from build123d import *

# Parameters (mm, degrees)
SKETCH1_R           = 10
BOSS_EXTRUDE1_DEPTH = 61
SKETCH3_W           = 66
SKETCH3_H           = 1.5
SKETCH4_W           = 45
SKETCH4_H           = 1.5
SKETCH5_W           = 25
SKETCH5_H           = 2.5
SKETCH6_W           = 39.5
SKETCH6_H           = 1
SKETCH7_W           = 25
SKETCH7_H           = 1.5
SKETCH8_W           = 1.1
SKETCH8_H           = 0.6
SKETCH9_W           = 1.1
SKETCH9_H           = 0.65
SKETCH10_W          = 1.1
SKETCH10_H          = 0.65


with BuildPart() as part:
    # Sketch1 → Boss-Extrude1 (new, symmetric)
    with BuildSketch(Plane.XY):
        with Locations(Location((0, 0, 0), (0, 0, 180))):
            Circle(SKETCH1_R)
    extrude(amount=BOSS_EXTRUDE1_DEPTH, both=True)

    # Sketch3 → Cut-Revolve1 (revolve, cut)
    with BuildSketch(Plane(origin=(0, 0, 0), x_dir=(0, 0, -1), z_dir=(1, 0, 0)), mode=Mode.PRIVATE) as cut_revolve1_sk:
        with Locations((28, 9.25)):
            Rectangle(SKETCH3_W, SKETCH3_H)
    revolve(cut_revolve1_sk.sketch.rotate(Axis((0, 0, 0), (0, 0, -1)), 270), axis=Axis((0, 0, 0), (0, 0, -1)), mode=Mode.SUBTRACT)

    # Sketch4 → Cut-Revolve2 (revolve, cut)
    with BuildSketch(Plane(origin=(0, 0, 0), x_dir=(0, 0, -1), z_dir=(1, 0, 0)), mode=Mode.PRIVATE) as cut_revolve2_sk:
        with Locations((-38.5, 9.25)):
            Rectangle(SKETCH4_W, SKETCH4_H)
    revolve(cut_revolve2_sk.sketch.rotate(Axis((0, 0, 0), (0, 0, 1)), 90), axis=Axis((0, 0, 0), (0, 0, 1)), mode=Mode.SUBTRACT)

    # Sketch5 → Cut-Revolve3 (revolve, cut)
    with BuildSketch(Plane(origin=(0, 0, 0), x_dir=(0, 0, -1), z_dir=(1, 0, 0)), mode=Mode.PRIVATE) as cut_revolve3_sk:
        with Locations((-48.5, 7.25)):
            Rectangle(SKETCH5_W, SKETCH5_H)
    revolve(cut_revolve3_sk.sketch.rotate(Axis((0, 0, 0), (0, 0, 1)), 90), axis=Axis((0, 0, 0), (0, 0, 1)), mode=Mode.SUBTRACT)

    # Sketch6 → Cut-Revolve4 (revolve, cut)
    with BuildSketch(Plane(origin=(0, 0, 0), x_dir=(0, 0, -1), z_dir=(1, 0, 0)), mode=Mode.PRIVATE) as cut_revolve4_sk:
        with Locations((41.25, 8)):
            Rectangle(SKETCH6_W, SKETCH6_H)
    revolve(cut_revolve4_sk.sketch.rotate(Axis((0, 0, 0), (0, 0, -1)), 90), axis=Axis((0, 0, 0), (0, 0, -1)), mode=Mode.SUBTRACT)

    # Sketch7 → Cut-Revolve5 (revolve, cut)
    with BuildSketch(Plane(origin=(0, 0, 0), x_dir=(0, 0, -1), z_dir=(1, 0, 0)), mode=Mode.PRIVATE) as cut_revolve5_sk:
        with Locations((48.5, 6.75)):
            Rectangle(SKETCH7_W, SKETCH7_H)
    revolve(cut_revolve5_sk.sketch.rotate(Axis((0, 0, 0), (0, 0, -1)), 90), axis=Axis((0, 0, 0), (0, 0, -1)), mode=Mode.SUBTRACT)

    # Sketch8 → Cut-Revolve6 (revolve, cut)
    with BuildSketch(Plane(origin=(0, 0, 0), x_dir=(0, 0, -1), z_dir=(1, 0, 0)), mode=Mode.PRIVATE) as cut_revolve6_sk:
        with Locations((30.95, 7.2)):
            Rectangle(SKETCH8_W, SKETCH8_H)
    revolve(cut_revolve6_sk.sketch.rotate(Axis((0, 0, 0), (0, 0, -1)), 90), axis=Axis((0, 0, 0), (0, 0, -1)), mode=Mode.SUBTRACT)

    # Sketch9 → Cut-Revolve7 (revolve, cut)
    with BuildSketch(Plane(origin=(0, 0, 0), x_dir=(0, 0, -1), z_dir=(1, 0, 0)), mode=Mode.PRIVATE) as cut_revolve7_sk:
        with Locations((5.45, 8.175)):
            Rectangle(SKETCH9_W, SKETCH9_H)
    revolve(cut_revolve7_sk.sketch.rotate(Axis((0, 0, 0), (0, 0, -1)), 90), axis=Axis((0, 0, 0), (0, 0, -1)), mode=Mode.SUBTRACT)

    # Sketch10 → Cut-Revolve8 (revolve, cut)
    with BuildSketch(Plane(origin=(0, 0, 0), x_dir=(0, 0, -1), z_dir=(1, 0, 0)), mode=Mode.PRIVATE) as cut_revolve8_sk:
        with Locations((-33.45, 8.175)):
            Rectangle(SKETCH10_W, SKETCH10_H)
    revolve(cut_revolve8_sk.sketch.rotate(Axis((0, 0, 0), (0, 0, 1)), 90), axis=Axis((0, 0, 0), (0, 0, 1)), mode=Mode.SUBTRACT)


solid = part.part
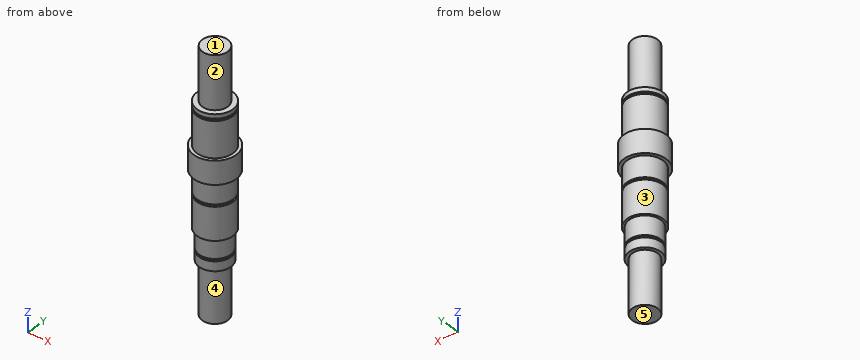
Can you work these out from the model? Positions are in its coordinate system, mm. Face numbers are marked on the shaded views. A direction names the side the tool comes from. Give positions to 0.01 mm unless a question says otherwise; leave off trailing zeros. Order: outer loops, then holes, each group sorted by start corner. A loop starts at its lowest first (then second) coordinate and runs counter-clockwise, first axis right, second up. Notation, with made-up numbers: M 87,40 L 115,40 A23 ccw 115,72 Z; hole C -22,30.25 d2. An arc over 180 degrees is marked long. Use one line per item in the form item = value.
Item 1: For the marked faces 1, 2 and 3, which set-ups out of +Z, -Z, +X, -X, +Y, -Y let a thin tool reach every point of the face, with its end or its side?
Values follow:
face_1 = +Z, +X, -X, +Y, -Y
face_2 = +Z
face_3 = -Z
Item 2: If we section it at A-A, the plane z = 52: Write out the boundary of the cut face in (x, y), and give its area (3 significant figures).
Values follow:
outline = C 0,0 d12
area = 113 mm^2
Item 3: If I drill on line 1 along Z through (x, y) = (7.5, -3); line 2 along Y through (x, z) = (-6, 24); line 3 along Z through (x, y) = (5, 3.75), over which ranges is the centre line in solid material (lowest first)? Write a range as [from, to].
Values follow:
line_1 = [-21.5, -6], [-4.9, 32.9], [34, 36]
line_2 = [-6.02, 6.02]
line_3 = [-36, 36]
Item 4: Will these pins go through, and if not, where does the flat tip stop? pin 1 Ø6 at (y, z) = (-3.5, -31.5) entering from -X; pin 2 Ø1.5 at (x, z) = (2, 18) entering from -Y; pin 3 Ø3 at (x, y) = (-4, 7) entering from +Z; pin 4 Ø1 at (x, y) = (6, 1) entering from -Z.
Values follow:
pin_1 = -7.48
pin_2 = -8.41
pin_3 = 36
pin_4 = -61
Item 5: If we section it at B-B, the plane z = -27: Write out the boundary of the cut face in (x, y).
Values follow:
outline = C 0,0 d15
Item 6: Thinking about a two-plate mould opening in X: for the marked faces 4 and 5, which applies, pulls with the +X half, pulls with the -X half, needs draft (parallel to the pull), parting line crosses it, or undercut?
Values follow:
face_4 = parting line crosses it
face_5 = needs draft
